Source: CAD feature listing. Evaluate the final solid. Frame: model axes, mm. A direction names the side the tool comes from. Give positions to 0.01 mm unless a question says otherwise; leave off trailing zeros. Loops run counter-clockwise (first coordinate to the right, second up) from the corner with the lowest first, then second, coordinate; pieces in that order, holes last. Notation, with made-up numbers: (-17.5, 46) -> (-2.5, 46) arc R23 ccw to (-2.5, 80) -> close; hole circle Ø1 at (11, 26). An arc over 180 degrees is marked (long way). Return JSON: item names as keys, results as strings. Group by question number.
(1) Cut plane A-A on z = -15.5. Return loops of the section in (x, y).
(2) Cut plane D-D on z = 14. Return loops of the section in (x, y), then the cut area to 3 significant figures.
(3) Access query for faces 1 (the face through (0, -17, 0)), 2 (the face through (2.66, 1.97, -9.41)), 3 (the face through (3, -2, -15)). Directions: +Z, -Z, +X, -X, +Y, -Y. A direction counts if a zero-diameter tool reaches every point of the face in a straight line with its end or side. Return the directions, or none.
(4) Pin query (flat end, axial travel): pin 1 (8 mm diameter, centred on x = 0, z = -13.94, fed in from +Y); pin 2 (1 mm diameter, centred on x = 6.5, y = -9.5, fed in from -Z); pin 3 (3 mm diameter, centred on x = 4.5, y = 0, fed in from -Z). Return the tip coordinate at first contact, or that it passes through.
(5) Ray query, line 1 (Y direction, x = -1.5, z = -10.5); line 2 (X direction, y = -15.75, z = -17); line 3 (X direction, y = 1.5, z = -8.5). Return the intervals inside material, ascending. Write a range as from..to.
(6) Cut plane B-B on x = 1.5. Return loops of the section in (y, z), then the cut area to 3 significant figures.
(7) Draft query along Z for faces 4 (the face through (-5.25, 2, -14)), 5 (the face through (8.024, -3.96, 22.994)), 6 (the face through (0.65, -0.986, -16.866)), 7 (the face through (-7.954, -3.737, -22.985)). Return one class per face: released by +Z, released by -Z, zero draft, split by the parting line, or undercut.
(8) Cut plane C-C on x = 4.5. Return loops of the section in (y, z).
Autodesk Inventor part; units mm, degrees
ref_plane "YZ Plane" through (0, 0, 0) normal (1, 0, 0) x (0, 1, 0)
ref_plane "XZ Plane" through (0, 0, 0) normal (0, 1, 0) x (-1, 0, 0)
ref_plane "XY Plane" through (0, 0, 0) normal (0, 0, 1) x (1, 0, 0)
sketch "Skizze1" plane through (0, 0, 0) normal (0, 1, 0) x (-1, 0, 0)
  line L0 (-10, 25) -> (10, 25)
  line L1 (10, 25) -> (10, -25)
  line L2 (10, -25) -> (-10, -25)
  line L3 (-10, -25) -> (-10, 25)
  line L4 (-10, 25) -> (10, -25) construction
  line L5 (10, 25) -> (-10, -25) construction
  line L6 (0, -20) -> (-5.25, -16.9689)
  line L7 (-5.25, -16.9689) -> (-5.25, -10.9067)
  line L8 (-5.25, -10.9067) -> (0, -7.8756)
  line L9 (0, -7.8756) -> (5.25, -10.9067)
  line L10 (5.25, -10.9067) -> (5.25, -16.9689)
  line L11 (5.25, -16.9689) -> (0, -20)
  circle A0 centre (0, -13.9378) radius 3
  circle A1 centre (0, -13.9378) radius 6.0622
  point P0 (0, 0)
  point P1 (0, 0)
  dimension "d0" = 10.5
  dimension "d1" = 20
  dimension "d2" = 50
  dimension "d3" = 5
  dimension "d6" = 6
extrude "Extrusion1" add sketch "Skizze1" against normal blind 2 contours L0 L1 L2 L3 | A1 L6 | L6 L7 L8 L9 L10 L11 | L11 A1 | A1 L7 | L10 A1 | A1 L8 | L9 A1
extrude "Extrusion2" add sketch "Skizze1" along normal blind 4 contours L0 L1 L2 L3 | A1 L6 | L11 A1 | A1 L7 | L10 A1 | A1 L8 | L9 A1
extrude "Extrusion3" add sketch "Skizze1" against normal blind 17 contours L0 L1 L2 L3
sketch "Skizze2" plane through (0, 0, 0) normal (1, 0, 0) x (0, 1, 0)
  line L0 (0, -10.9378) -> (-2, -10.9378)
  line L1 (-2, -10.9378) -> (-2, -7.8756)
  line L2 (-2, -7.8756) -> (-17, -7.8756)
  line L3 (-17, -7.8756) -> (-17, 25)
  line L4 (-17, 25) -> (4, 25)
  line L5 (4, 25) -> (4, -7.8756)
  line L6 (4, -7.8756) -> (0, -7.8756)
  line L7 (0, -7.8756) -> (0, -10.9378)
  line L8 (-2, -16.9378) -> (0, -16.9378)
  line L9 (0, -16.9378) -> (0, -20)
  line L10 (0, -20) -> (4, -20)
  line L11 (4, -20) -> (4, -25)
  line L12 (4, -25) -> (-17, -25)
  line L13 (-17, -25) -> (-17, -20)
  line L14 (-17, -20) -> (-2, -20)
  line L15 (-2, -20) -> (-2, -16.9378)
  line L16 (-12, 25) -> (4, 22.1788)
  line L17 (4, 25) -> (4, 22.1788)
  line L18 (4, 25) -> (-12, 25)
  line L19 (4, -22.1788) -> (4, -25)
  line L20 (4, -22.1788) -> (-12, -25)
  line L21 (4, -25) -> (-12, -25)
  point P0 (0, 0)
  dimension "d12" = 5
  dimension "d13" = 10
  dimension "d14" = 10
extrude "Extrusion4" cut sketch "Skizze2" along normal through all both and the other way through all contours L16 L4 L5 | L11 L12 L20
sketch "Skizze3" plane through (0, 0, 0) normal (0, 0, 1) x (1, 0, 0)
  line L0 (-10, 4) -> (10, 4)
  line L1 (10, 4) -> (10, -17)
  line L2 (10, -17) -> (-10, -17)
  line L3 (-10, -17) -> (-10, 4)
  line L4 (-7.1788, 4) -> (-10, 4)
  line L5 (-10, -12) -> (-10, 4)
  line L6 (-10, -12) -> (-7.1788, 4)
  line L7 (7.1788, 4) -> (10, 4)
  line L8 (10, 4) -> (10, -12)
  line L9 (10, -12) -> (7.1788, 4)
  point P0 (0, 0)
  dimension "d17" = 10
  dimension "d18" = 10
  dimension "d19" = 5
extrude "Extrusion5" cut sketch "Skizze3" along normal through all both and the other way through all contours L0 L6 L3 | L0 L1 L9
fillet "Rundung1" radius 2 8 edges at (8.5894, -4, 23.5894) (10, -14.5, 25) (-8.5894, -4, 23.5894) (-10, -14.5, 25) (-8.5894, -4, -23.5894) (-10, -14.5, -25) (8.5894, -4, -23.5894) (10, -14.5, -25)
equation "\"d18\" = d17"
equation "\"d19\" = d12"
properties part number "Verschluss_Knauf"
Answers:
{
 "1": {"outline": "(-10, -17) -> (-5.86, -17) -> (-5.86, -2) -> (-2.56, -2) -> (-2.56, 0) -> (-5.25, 0) -> (-5.25, 4) -> (-7.18, 4) -> (-10, -12) -> close; (2.56, -2) -> (5.86, -2) -> (5.86, -17) -> (10, -17) -> (10, -12) -> (7.18, 4) -> (5.25, 4) -> (5.25, 0) -> (2.56, 0) -> close"},
 "2": {"outline": "(-10, -17) -> (10, -17) -> (10, -12) -> (7.18, 4) -> (-7.18, 4) -> (-10, -12) -> close", "area": "375 mm²"},
 "3": {"face 1": "+Z, -Z, +X, -X, -Y", "face 2": "+Y", "face 3": "-Y"},
 "4": {"pin 1": "y = 0", "pin 2": "z = -24.65", "pin 3": "z = -23.15"},
 "5": {"line 1": "-2..0", "line 2": "-10..-5.23, 5.23..10", "line 3": "-7.62..-1.08, 1.08..7.62"},
 "6": {"outline": "(-17, -25) -> (-12, -25) -> (4, -22.18) -> (4, -19.13) -> (0, -19.13) -> (0, -16.54) -> (-2, -16.54) -> (-2, -19.81) -> (-17, -19.81) -> close; (-17, -8.06) -> (-2, -8.06) -> (-2, -11.34) -> (0, -11.34) -> (0, -8.74) -> (4, -8.74) -> (4, 22.18) -> (-12, 25) -> (-17, 25) -> close", "area": "777 mm²"},
 "7": {"face 4": "undercut", "face 5": "released by +Z", "face 6": "undercut", "face 7": "released by -Z"},
 "8": {"outline": "(-17, -25) -> (-12, -25) -> (4, -22.18) -> (4, -17.4) -> (0, -17.4) -> (0, -10.47) -> (4, -10.47) -> (4, 22.18) -> (-12, 25) -> (-17, 25) -> (-17, -9.88) -> (-2, -9.88) -> (-2, -18) -> (-17, -18) -> close"}
}
